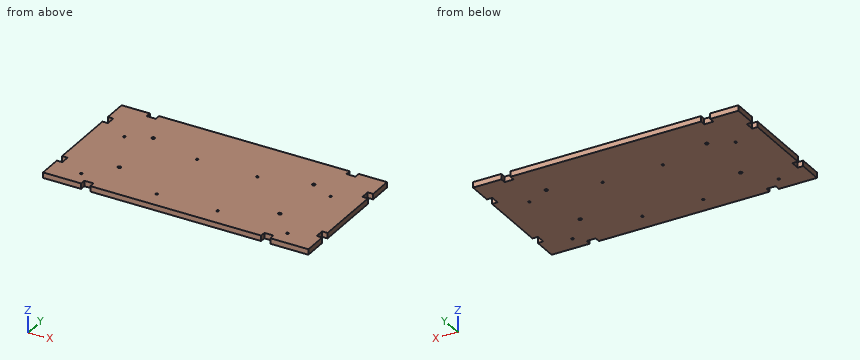
```python
from build123d import *

# Parameters (mm, degrees)
F0_R     = 1.25
F0_R_2   = 1.75
F1_DEPTH = 6


# Not quite as in the source:
# - a feature names something its author has since deleted; it is built from what else it names


with BuildPart() as f1:
    # F0 (on Top) → F1 (new body)
    with BuildSketch(Plane.XY):
        Polygon((145.5019380654, -28.2040820618), (145.5019380654, 47.7959179382), (139.5019380654, 47.7959179382), (139.5019380654, 57.7961117593), (145.5019380654, 57.7961117593), (145.4994183911, 83.7961116372), (114.4994185367, 83.7931074102), (114.5, 77.7931074384), (104.5, 77.7931074384), (104.5, 83.793107429), (0, 83.793107429), (-104.5, 83.793107429), (-104.5, 77.7931074384), (-114.5, 77.7931074384), (-114.4994185367, 83.7931074102), (-145.4994183911, 83.7961116372), (-145.5019380654, 57.7961117593), (-139.5019380654, 57.7961117593), (-139.5019380654, 47.7959179382), (-145.5019380654, 47.7959179382), (-145.5019380654, -28.2040820618), (-139.5019380654, -28.2040820618), (-139.5019380654, -38.2040820618), (-145.5019380652, -38.2041248082), (-145.5019380652, -64.2040820618), (-103.7128691326, -64.2040817458), (-103.7128691326, -58.2040817458), (-93.6722421218, -58.2040816699), (-93.6722421218, -64.2042880704), (-4.2916e-06, -64.2042880704), (93.6722421218, -64.2042880704), (93.6722421218, -58.2040816699), (103.7128691326, -58.2040817458), (103.7128691326, -64.2040817458), (145.5019380652, -64.2040820618), (145.5019380652, -38.2041248082), (139.5019380654, -38.2040820618), (139.5019380654, -28.2040820618), align=None)
        with Locations((-113.03, -48.0000058421)):
            Circle(F0_R, mode=Mode.SUBTRACT)
        with Locations((-31.75, -45.4600058421)):
            Circle(F0_R, mode=Mode.SUBTRACT)
        with Locations((-88, -19.2042880704)):
            Circle(F0_R_2, mode=Mode.SUBTRACT)
        with Locations((34.29, -44.1900058421)):
            Circle(F0_R, mode=Mode.SUBTRACT)
        with Locations((113.03, -47.8810681991)):
            Circle(F0_R, mode=Mode.SUBTRACT)
        with Locations((88, -19.2042880704)):
            Circle(F0_R_2, mode=Mode.SUBTRACT)
        with Locations((-113.03, 33.2799941579)):
            Circle(F0_R, mode=Mode.SUBTRACT)
        with Locations((-88, 44.7957119296)):
            Circle(F0_R_2, mode=Mode.SUBTRACT)
        with Locations((-31.75, 30.7399941579)):
            Circle(F0_R, mode=Mode.SUBTRACT)
        with Locations((34.29, 30.7399941579)):
            Circle(F0_R, mode=Mode.SUBTRACT)
        with Locations((88, 44.7957119296)):
            Circle(F0_R_2, mode=Mode.SUBTRACT)
        with Locations((113.03, 33.3989318009)):
            Circle(F0_R, mode=Mode.SUBTRACT)
    extrude(amount=F1_DEPTH)


solid = f1.part
```
CAD build for the part. Positions are in the model's coordinates, mm. Round coordinates to 2 decimals unless told otherwise and drop trailing zeros. Order: outer loops, then holes, each group sorted by start corner. A loop starts at its lowest first (then second) coordinate and runs counter-clockwise, first axis right, second up.
Q1. Wall check: L1, parallel to Y at x = -88, z = 1.95; L2, parallel to Y at x = -113.03, z = 2.75; L3, parallel to Y at x = 4, z = 4.4. Give the ranges that are in metal, low to high.
Q2. Drop flat-ended pins along their axis: pin 1 (4 mm diameter, centred on x = 113.03, y = -47.88, fed in from +Z); pin 2 (1.8 mm diameter, centred on y = 80.5, z = 1.5, fed in from +X). Give the stop position or say it passes through.
Q3. Slice it at A-A (x = 96.5). Write the cut outline in (y, z).
Results below:
1. L1: y = -64.2 to -20.95, -17.45 to 43.05, 46.55 to 83.79
1. L2: y = -64.2 to -49.25, -46.75 to 32.03, 34.53 to 77.79
1. L3: y = -64.2 to 83.79
2. pin 1: stops at z = 6
2. pin 2: stops at x = 145.5
3. outline: (-58.2, 0) - (83.79, 0) - (83.79, 6) - (-58.2, 6) - close
